Can you work these out from the model? Positions are in its coordinate system, mm. A direction names the side the tool comes from. Round coordinates to 2 decimals unless told otherwise and drop trailing zeros. Write each loop counter-clockwise with the first axis right and the second up, starting at its lowest first coordinate (ties: lowest second). Pieces come first, ordered by that corner, then holes.
Q1. If we section it at A-A (z = 45): Please give me the cut outline in (x, y), plus the area to 3 significant figures.
Q2. If we section it at B-B (x = 0): Please give me the cut outline in (y, z).
Q3. Please list where these lines run through material, in increasing order: line 1 along Y through (x, z) = (0, 53.5); line 2 along Y through (x, z) = (-10, 63.5); line 3 along X through (y, z) = (0, 56).
Q4. We'd pull the mould along X, two halves only. Please class faces 1 (the cylindrical face through (-19.743, -27.086, 49.72)), 2 (the cylindrical face through (-12.67, 4.25, 33.12)), 3 (the cylindrical face through (22.1, -5.3, 49.7)): +X half, -X half, draft (parallel to the pull), parting line (faces both ways), or undercut.
Q5. If we section it at C-C (y = -22): Please give me the cut outline in (x, z).
Q6. I'm going to push flat-ended pins straight in: pin 1 Ø12 at (x, z) = (0.5, 61) entering from -Y; pin 2 Ø2 at (x, z) = (1.5, 42.5) entering from -Y; pin 3 Ø8 at (x, z) = (-9, 36.5) entering from -Y. Where does each tip first touch, or does it pass through?
Q7. For faces 4 (the cylindrical face through (8.314, -3.447, 51.241)), 5 (the flat face through (-11, 3, 70)), 6 (the cylindrical face through (-11.45, 0.15, 63.29)), which set-ups out of +Z, -Z, +X, -X, +Y, -Y let a thin tool reach every point of the face, with its end or its side?
from build123d import *

# Parameters (mm, degrees)
SKETCH1_R               = 9
BOSS_EXTRUDE1_DEPTH     = 70
SKETCH2_R               = 2.5
CUT_EXTRUDE1_DEPTH      = 5
CUT_EXTRUDE2_REACH      = 90.987
CUT_EXTRUDE2_END_RADIUS = 9
SKETCH3_R               = 1.75
CIRPATTERN1_COUNT       = 3
SKETCH5_W               = 24.568161226
SKETCH5_H               = 25
SKETCH6_R               = 9
BOSS_EXTRUDE2_DEPTH     = 5
SKETCH8_R               = 9
BOSS_EXTRUDE3_DEPTH     = 3
CUT_EXTRUDE3_REACH      = 83.112
SKETCH9_R               = 1.875
SKETCH11_R              = 4
CUT_EXTRUDE4_DEPTH      = 3
CUT_EXTRUDE5_DEPTH      = 82.111701173
CUT_EXTRUDE5_DEPTH_BACK = 82.111701173
SKETCH12_W              = 65.170629785
SKETCH12_H              = 33.219663289
CUT_EXTRUDE6_REACH      = 89.673
CUT_EXTRUDE6_END_RADIUS = 9
SKETCH13_R              = 5


with BuildPart() as part:
    # Sketch1 → Boss-Extrude1 (new body)
    with BuildSketch(Plane.XY):
        with BuildLine():
            Line((-23.6546385, -16.539669722), (-13.23734813, 25.649078182))
            ThreePointArc((-13.23734813, 25.649078182), (-5.029445343, 33.138647287), (5.031042671, 28.421667909))
            Line((5.031042671, 28.421667909), (20.916771438, 2.118648772))
            ThreePointArc((20.916771438, 2.118648772), (22.065215706, -5.448366461), (17.526600651, -11.611126974))
            Line((17.526600651, -11.611126974), (-8.776418486, -27.496855741))
            ThreePointArc((-8.776418486, -27.496855741), (-19.876207308, -26.988917124), (-23.6546385, -16.539669722))
        make_face()
        Circle(SKETCH1_R, mode=Mode.SUBTRACT)
    extrude(amount=BOSS_EXTRUDE1_DEPTH)

    # Sketch2 → Cut-Extrude1 (cut)
    with BuildSketch(Plane(origin=(9.822624711, -16.263949206, 0), x_dir=(0.8559973266359324, 0.5169802479709809, 0), z_dir=(0.5169802479709809, -0.8559973266359324, 0))):
        with Locations((0, 65)):
            Circle(SKETCH2_R)
    cut_extrude1 = extrude(amount=-CUT_EXTRUDE1_DEPTH, mode=Mode.SUBTRACT)

    # Cut-Extrude2: up to this cylinder (the profile starts outside it)
    cut_extrude2_end = Plane(origin=(0, 0, 65), z_dir=(0, 0, -1)) * Cylinder(CUT_EXTRUDE2_END_RADIUS, 200.974, mode=Mode.PRIVATE)
    # Sketch3 → Cut-Extrude2 (cut, up to the surface)
    with BuildSketch(Plane(origin=(7.237723472, -11.983962573, 0), x_dir=(0.8559973266359324, 0.5169802479709809, 0), z_dir=(0.5169802479709809, -0.8559973266359324, 0)), mode=Mode.PRIVATE) as cut_extrude2_sk1:
        with Locations((0, 65)):
            Circle(SKETCH3_R)
    cut_extrude2_tool1 = extrude(cut_extrude2_sk1.sketch, amount=-CUT_EXTRUDE2_REACH, mode=Mode.PRIVATE) - cut_extrude2_end
    cut_extrude2 = cut_extrude2_tool1.solids().sort_by_distance((7.237723, -11.983963, 65))[0]
    add(cut_extrude2, mode=Mode.SUBTRACT)

    # CirPattern1: Cut-Extrude1, Cut-Extrude2 ×3 about axis
    cirpattern1_axis = Axis((0, 0, 0), (0, 0, 1))
    add([cut_extrude1.rotate(cirpattern1_axis, i * 360 / CIRPATTERN1_COUNT) for i in range(1, CIRPATTERN1_COUNT)], mode=Mode.SUBTRACT)
    add([cut_extrude2.rotate(cirpattern1_axis, i * 360 / CIRPATTERN1_COUNT) for i in range(1, CIRPATTERN1_COUNT)], mode=Mode.SUBTRACT)

    # Sketch5 → Cut-Revolve1 (revolve, cut)
    with BuildSketch(Plane(origin=(0, 0, 0), x_dir=(1, 0, 0), z_dir=(0, 1, 0)), mode=Mode.PRIVATE) as cut_revolve1_sk:
        with Locations((-12.284080613, -17.5)):
            Rectangle(SKETCH5_W, SKETCH5_H)
    revolve(cut_revolve1_sk.sketch.rotate(Axis((0, 0, 0), (0, 0, 1)), 180), axis=Axis((0, 0, 0), (0, 0, 1)), mode=Mode.SUBTRACT)

    # Sketch6 → Boss-Extrude2 (add)
    with BuildSketch(Plane(origin=(0, 0, 0), x_dir=(-1, 0, 0), z_dir=(0, 0, -1))):
        with Locations(Location((0, 0, 0), (0, 0, 180))):
            Circle(SKETCH6_R)
    extrude(amount=-BOSS_EXTRUDE2_DEPTH)

    # Sketch8 → Boss-Extrude3 (add)
    with BuildSketch(Plane(origin=(0, 0, 30), x_dir=(-1, 0, 0), z_dir=(0, 0, -1))):
        Circle(SKETCH8_R)
    extrude(amount=-BOSS_EXTRUDE3_DEPTH)

    # Sketch9 → Cut-Extrude3 (cut, up to next)
    with BuildSketch(Plane(origin=(0, 0, 0), x_dir=(-1, 0, 0), z_dir=(0, 0, -1)), mode=Mode.PRIVATE) as cut_extrude3_sk1:
        with Locations((0, 8)):
            Circle(SKETCH9_R)
    cut_extrude3_tool1 = extrude(cut_extrude3_sk1.sketch, amount=-CUT_EXTRUDE3_REACH, mode=Mode.PRIVATE) & part.part
    # Sketch9 → Cut-Extrude3 (cut, up to next)
    with BuildSketch(Plane(origin=(0, 0, 0), x_dir=(-1, 0, 0), z_dir=(0, 0, -1)), mode=Mode.PRIVATE) as cut_extrude3_sk2:
        with Locations((8, 0)):
            Circle(SKETCH9_R)
    cut_extrude3_tool2 = extrude(cut_extrude3_sk2.sketch, amount=-CUT_EXTRUDE3_REACH, mode=Mode.PRIVATE) & part.part
    # Sketch9 → Cut-Extrude3 (cut, up to next)
    with BuildSketch(Plane(origin=(0, 0, 0), x_dir=(-1, 0, 0), z_dir=(0, 0, -1)), mode=Mode.PRIVATE) as cut_extrude3_sk3:
        with Locations((0, -8)):
            Circle(SKETCH9_R)
    cut_extrude3_tool3 = extrude(cut_extrude3_sk3.sketch, amount=-CUT_EXTRUDE3_REACH, mode=Mode.PRIVATE) & part.part
    # Sketch9 → Cut-Extrude3 (cut, up to next)
    with BuildSketch(Plane(origin=(0, 0, 0), x_dir=(-1, 0, 0), z_dir=(0, 0, -1)), mode=Mode.PRIVATE) as cut_extrude3_sk4:
        with Locations((-8, 0)):
            Circle(SKETCH9_R)
    cut_extrude3_tool4 = extrude(cut_extrude3_sk4.sketch, amount=-CUT_EXTRUDE3_REACH, mode=Mode.PRIVATE) & part.part
    add(cut_extrude3_tool1.solids().sort_by_distance((0, 8, 0))[0], mode=Mode.SUBTRACT)
    add(cut_extrude3_tool2.solids().sort_by_distance((-8, 0, 0))[0], mode=Mode.SUBTRACT)
    add(cut_extrude3_tool3.solids().sort_by_distance((0, -8, 0))[0], mode=Mode.SUBTRACT)
    add(cut_extrude3_tool4.solids().sort_by_distance((8, 0, 0))[0], mode=Mode.SUBTRACT)

    # Sketch11 → Cut-Extrude4 (cut)
    with BuildSketch(Plane(origin=(0, 0, 0), x_dir=(-1, 0, 0), z_dir=(0, 0, -1))):
        Circle(SKETCH11_R)
    extrude(amount=-CUT_EXTRUDE4_DEPTH, mode=Mode.SUBTRACT)

    # Sketch12 → Cut-Extrude5 (cut, two sides: drawn at the far end of the back side and taken through both)
    with BuildSketch(Plane(origin=(0, 0, 0), x_dir=(1, 0, 0), z_dir=(0, 1, 0)).offset(-CUT_EXTRUDE5_DEPTH_BACK)):
        with Locations((1.843004816, -13.390168356)):
            Rectangle(SKETCH12_W, SKETCH12_H)
    extrude(amount=CUT_EXTRUDE5_DEPTH + CUT_EXTRUDE5_DEPTH_BACK, mode=Mode.SUBTRACT)

    # Cut-Extrude6: up to this cylinder (the profile starts outside it)
    cut_extrude6_end = Plane(origin=(0, 0, 38), z_dir=(0, 0, -1)) * Cylinder(CUT_EXTRUDE6_END_RADIUS, 198.346, mode=Mode.PRIVATE)
    # Sketch13 → Cut-Extrude6 (cut, up to the surface)
    with BuildSketch(Plane(origin=(-18.445993315, 4.55470423, 0), x_dir=(0, 0, 1), z_dir=(-0.9708417534216062, 0.23972127526204579, 0)), mode=Mode.PRIVATE) as cut_extrude6_sk1:
        with Locations(Location((38, 0, 0), (0, 0, 270))):
            Circle(SKETCH13_R)
    cut_extrude6_tool1 = extrude(cut_extrude6_sk1.sketch, amount=-CUT_EXTRUDE6_REACH, mode=Mode.PRIVATE) - cut_extrude6_end
    add(cut_extrude6_tool1.solids().sort_by_distance((-18.445993, 4.554704, 38))[0], mode=Mode.SUBTRACT)


solid = part.part
A:
1. outline: (-23.65, -16.54) arc R10 ccw to (-8.78, -27.5) - (17.53, -11.61) arc R10 ccw to (20.92, 2.12) - (5.03, 28.42) arc R10 ccw to (-13.24, 25.65) - close; hole circle Ø18 at (0, 0)
1. area: 1,580 mm2
2. outline: (-22.2, 30) - (32.61, 30) - (32.61, 70) - (9, 70) - (9, 33) - (-9, 33) - (-9, 70) - (-22.2, 70) - close
3. line 1: y = -22.2 to -9, 9 to 32.61
3. line 2: y = -28.13 to -1.1, 0.7 to 30.88
3. line 3: x = -19.57 to -9, 9 to 21.88
4. face 1: parting line
4. face 2: undercut
4. face 3: +X half
5. outline: (-23.47, 30) - (0.33, 30) - (0.33, 70) - (-23.47, 70) - close
6. pin 1: stops at y = -25.52
6. pin 2: stops at y = -21.89
6. pin 3: stops at y = -28.89
7. face 4: +Z
7. face 5: +Z, +X, -X, +Y, -Y
7. face 6: none
